Can you work these out from the drawing? Everything is in mm from the part's minimum corner. A direction names the side the tool comes from. Round coordinates to 2 decimals unless told otherwise and drop trailing zeros. Write each loop counter-clockwise with the first axis right and the second up, starting at its lowest first coordinate (ties: lowest second). Pieces come first, ordered by that corner, then holes.
Q1. If we section it at A-A (x = 35): Please give me the cut outline in (y, z).
Q2. If we section it at B-B (y = 5): Please give me the cut outline in (x, z), plus the area to 3 significant figures.
Q3. We'd pull the mould along Z, two halves only. Please class the marked faces 1, 2, 3 and 4: +Z half, -Z half, draft (parallel to the pull), parting line (faces both ways), or undercut.
Q4. For the marked faces 5 and 6, which set-ups out of +Z, -Z, +X, -X, +Y, -Y let a thin tool reach every point of the face, with its end or its side?
Q5. I'm going to push flat-ended pins straight in: pin 1 Ø3 at (y, z) = (15.5, 14) entering from +X; pin 2 Ø3 at (x, z) = (12.5, 50) entering from -Y; pin 3 Ø8 at (x, z) = (8, 63.5) entering from -Y. Where does each tip first touch, or does it pass through?
Q6. Please list where these lines run through material, in increasing order: line 1 along Z through (x, y) = (45, 59); line 2 along X through (y, z) = (35.5, 88) (3 decimals); line 3 along Y through (x, z) = (36, 85.5).
Q7. If we section it at D-D (z = 72): Please give me the cut outline in (x, y), plus the area to 3 significant figures.
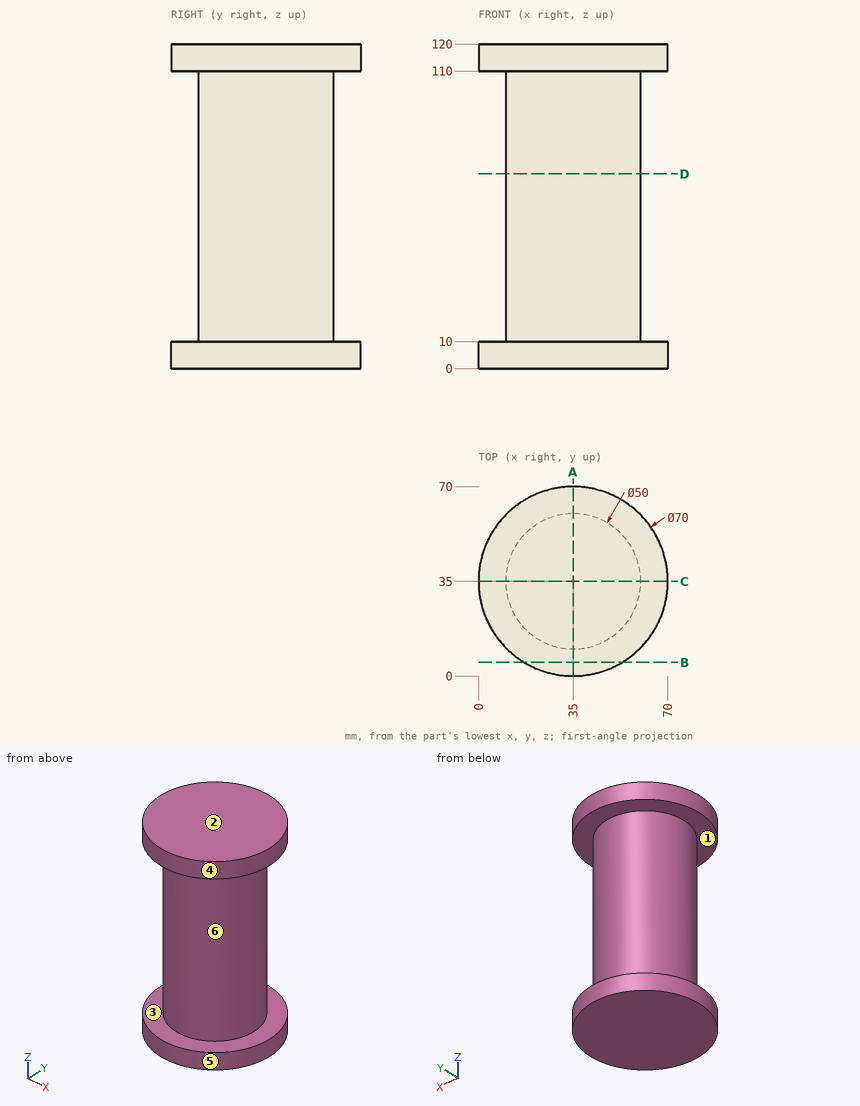
A:
1. outline: (0, 0) - (70, 0) - (70, 10) - (60, 10) - (60, 110) - (70, 110) - (70, 120) - (0, 120) - (0, 110) - (10, 110) - (10, 10) - (0, 10) - close
2. outline: (16.97, 0) - (53.03, 0) - (53.03, 10) - (16.97, 10) - close; (16.97, 110) - (53.03, 110) - (53.03, 120) - (16.97, 120) - close
2. area: 721 mm2
3. face 1: undercut
3. face 2: +Z half
3. face 3: undercut
3. face 4: draft
4. face 5: +Z, -Z
4. face 6: none
5. pin 1: stops at x = 52.35
5. pin 2: stops at y = 21.44
5. pin 3: stops at y = 25.2
6. line 1: z = 0 to 10, 110 to 120
6. line 2: x = 10.005 to 59.995
6. line 3: y = 10.02 to 59.98
7. outline: circle Ø50 at (35, 35)
7. area: 1,960 mm2
